```python
from build123d import *

# Parameters (mm, degrees)
ESQUISSE1_R        = 19.06
BOSS_EXTRU_1_DEPTH = 8
BOSS_EXTRU_2_DEPTH = 3


with BuildPart() as part:
    # Esquisse1 → Boss.-Extru.1 (new body)
    with BuildSketch(Plane(origin=(0, 0, 0), x_dir=(1, 0, 0), z_dir=(0, 1, 0))):
        with Locations(Location((0, 0, 0), (0, 0, 270))):
            Circle(ESQUISSE1_R)
    extrude(amount=BOSS_EXTRU_1_DEPTH)

    # Esquisse2 → Boss.-Extru.2 (add)
    with BuildSketch(Plane(origin=(0, 8, 0), x_dir=(1, 0, 0), z_dir=(0, 1, 0))):
        Polygon((0, 3.1), (3.1, 3.1), (3.1, -3.1), (-3.1, -3.1), (-3.1, 3.1), align=None)
    extrude(amount=BOSS_EXTRU_2_DEPTH)


solid = part.part
```
For this review, take the finished solid that the model builds, in its own axes (mm). A direction names the side the tool comes from. Round coordinates to 2 decimals unless told otherwise and drop trailing zeros. Order: outer loops, then holes, each group sorted by start corner. A loop starts at its lowest first (then second) coordinate and runs counter-clockwise, first axis right, second up. Notation, with made-up numbers: (42.5, 57) -> (96.5, 57) arc R30 ccw to (96.5, 85) -> close; hole circle Ø5 at (58, 42). An arc over 180 degrees is marked (long way). Use a Markdown table: item, result.
Item 1: Take a section at D-D (x = 11.5). State the section outline as (y, z) points.
Resolved:
| item | result |
|---|---|
| outline | (0, -15.2) -> (8, -15.2) -> (8, 15.2) -> (0, 15.2) -> close |
Item 2: For pin 1 (1 mm diameter, centred on x = 9.5, y = 1.5, fed in from +Z); pin 2 (5 mm diameter, centred on x = 13.5, y = 9, fed in from -Z); pin 3 (1.5 mm diameter, centred on x = -1, y = 10, fed in from +Z), all flat-tipped, find the tip position at first contact; note any pin that passes through.
Resolved:
| item | result |
|---|---|
| pin 1 | stops at z = 16.8 |
| pin 2 | stops at z = -15.42 |
| pin 3 | stops at z = 3.1 |
Item 3: Take a section at B-B (z = 0). State the section outline as (x, y) points.
Resolved:
| item | result |
|---|---|
| outline | (-19.06, 0) -> (19.06, 0) -> (19.06, 8) -> (3.1, 8) -> (3.1, 11) -> (-3.1, 11) -> (-3.1, 8) -> (-19.06, 8) -> close |
Item 4: Take a section at A-A (x = 0). State the section outline as (y, z) points.
Resolved:
| item | result |
|---|---|
| outline | (0, -19.06) -> (8, -19.06) -> (8, -3.1) -> (11, -3.1) -> (11, 3.1) -> (8, 3.1) -> (8, 19.06) -> (0, 19.06) -> close |
Item 5: For line 1 along Y through (x, z) = (13, -11.5); line 2 along X through (y, z) = (9.25, 3); line 3 along Z through (x, y) = (-11, 4), list the stretches that pass through material, from the lowest coordinate up. Write a range as [from, to].
Resolved:
| item | result |
|---|---|
| line 1 | y = [0, 8] |
| line 2 | x = [-3.1, 3.1] |
| line 3 | z = [-15.57, 15.57] |
Item 6: Machinability: for faces 1 (the flat face through (-3.1, 9, 0)), 2 (the flat face through (3.1, 9, 0)), 3 (the flat face through (0, 9, 3.1)), 4 (the flat face through (0, 9, -3.1)), which of the approach directions +Z, -Z, +X, -X, +Y, -Y give a long, thin tool a straight path to every point of the face, cutting with its end or side? Answer none if there is none.
Resolved:
| item | result |
|---|---|
| face 1 | +Z, -Z, -X, +Y |
| face 2 | +Z, -Z, +X, +Y |
| face 3 | +Z, +X, -X, +Y |
| face 4 | -Z, +X, -X, +Y |
Item 7: Take a section at C-C (y = 6.5). State the section outline as (x, z) points, plus the area to 3 significant figures.
Resolved:
| item | result |
|---|---|
| outline | circle Ø38.12 at (0, 0) |
| area | 1,140 mm² |
